Part model, mm, in its own coordinate system. Round coordinates to 2 decimals unless told otherwise and drop trailing zeros. Loops run counter-clockwise (first coordinate to the right, second up) from the corner with the lowest first, then second, coordinate; pieces in that order, holes last.
from build123d import *

# Parameters (mm, degrees)
SKETCH1_R           = 20
BOSS_EXTRUDE1_DEPTH = 10
FILLET1_R           = 5
FILLET2_R           = 5
SKETCH2_R           = 1.5
CUT_EXTRUDE1_DEPTH  = 31.000000133


with BuildPart() as part:
    # Sketch1 → Boss-Extrude1 (new body)
    with BuildSketch(Plane.XY):
        Circle(SKETCH1_R)
    extrude(amount=BOSS_EXTRUDE1_DEPTH)

    # Fillet1
    fillet1_edges = [part.edges().sort_by_distance(p)[0] for p in [
        (-20, 0, 10),
    ]]
    fillet(fillet1_edges, radius=FILLET1_R)

    # Fillet2
    fillet2_edges = [part.edges().sort_by_distance(p)[0] for p in [
        (-20, 0, 0),
    ]]
    fillet(fillet2_edges, radius=FILLET2_R - 0.0001)  # a hair under: the kernel refuses the full size

    # Sketch2 → Cut-Extrude1 (cut, through all)
    with BuildSketch(Plane.XY.offset(10)):
        Circle(SKETCH2_R)
    extrude(amount=-CUT_EXTRUDE1_DEPTH, mode=Mode.SUBTRACT)


solid = part.part
1) Drop flat-ended pins along their axis: pin 1 Ø1 at (x, y) = (-2, 6) entering from -Z; pin 2 Ø5 at (x, z) = (3.5, 1.5) entering from -Y; pin 3 Ø4 at (y, z) = (6, 7.5) entering from +X; pin 4 Ø1 at (x, z) = (1.5, 5) entering from +Y (3 decimals). Give the stop position or say it passes through.
Values:
pin 1: stops at z = 0
pin 2: stops at y = -19.69
pin 3: stops at x = 19.34
pin 4: stops at y = 19.975
2) Mould opens along Y. For faces 1 (the face through (0, -3, 0)), 2 (the face through (-1.5, 0.07, 5.07)) say: released by +Y, released by -Y, zero draft, split by the parting line, or undercut.
Values:
face 1: zero draft
face 2: undercut
3) Slice it at C-C, the plane z = 9. Give the cut face in (x, y).
Values:
outline: circle Ø36 at (0, 0); hole circle Ø3 at (0, 0)
4) Wall check: line 1 along Y through (x, z) = (0, 4); line 2 along Y through (x, z) = (10.5, 5); line 3 along Y through (x, z) = (3, 8.25). Give the ranges that are in metal, low to high.
Values:
line 1: y = -19.9 to -1.5, 1.5 to 19.9
line 2: y = -17.02 to 17.02
line 3: y = -18.56 to 18.56
5) Slice it at D-D, the plane z = 3. Give the cut face in (x, y).
Values:
outline: circle Ø39.17 at (0, 0); hole circle Ø3 at (0, 0)
